```python
from build123d import *

# Parameters (mm, degrees)
SKETCH_1_W                  = 66
SKETCH_1_H                  = 56
EXTRUDE_1_DEPTH             = 2
SKETCH_2_R                  = 1.6
CUT_EXTRUDE_1_DEPTH         = 2
PATTERN_LINEAR_1_COUNT      = 2
PATTERN_LINEAR_1_PITCH      = 50
PATTERN_LINEAR_1_COUNT_DIR2 = 2
PATTERN_LINEAR_1_PITCH_DIR2 = 40
SKETCH_4_R                  = 1.6
CUT_EXTRUDE_2_DEPTH         = 2
SKETCH_5_W                  = 18
SKETCH_5_H                  = 14
CUT_EXTRUDE_3_DEPTH         = 2
SKETCH_7_W                  = 18
SKETCH_7_H                  = 14
CUT_EXTRUDE_4_DEPTH         = 2
SKETCH_8_W                  = 12.2
SKETCH_8_H                  = 6.6
CUT_EXTRUDE_5_DEPTH         = 2


with BuildPart() as part:
    # 草图1 → 凸台-拉伸1 (new body)
    with BuildSketch(Plane(origin=(0, 0, 0), x_dir=(1, 0, 0), z_dir=(0, 1, 0))):
        Rectangle(SKETCH_1_W, SKETCH_1_H)
    extrude(amount=EXTRUDE_1_DEPTH)

    # 草图2 → 切除-拉伸1 (cut)
    with BuildSketch(Plane(origin=(0, 2, 0), x_dir=(1, 0, 0), z_dir=(0, 1, 0))):
        with Locations(Location((-25, 20, 0), (0, 0, 270))):
            Circle(SKETCH_2_R)
    cut_extrude_1 = extrude(amount=-CUT_EXTRUDE_1_DEPTH, mode=Mode.SUBTRACT)

    # 阵列(线性)1: Cut-Extrude 1 2 × 2
    with Locations(*[(i * PATTERN_LINEAR_1_PITCH, 0, j * PATTERN_LINEAR_1_PITCH_DIR2) for i in range(PATTERN_LINEAR_1_COUNT) for j in range(PATTERN_LINEAR_1_COUNT_DIR2) if (i, j) != (0, 0)]):
        add(cut_extrude_1, mode=Mode.SUBTRACT)

    # 草图4 → 切除-拉伸2 (cut)
    with BuildSketch(Plane.XZ):
        with Locations(Location((-17.49998476, 20.00007874, 0), (0, 0, 270))):
            Circle(SKETCH_4_R)
        with Locations(Location((-7.49996444, 20.00007874, 0), (0, 0, 270))):
            Circle(SKETCH_4_R)
        with Locations(Location((2.49985522, 19.999735839, 0), (0, 0, 270))):
            Circle(SKETCH_4_R)
    extrude(amount=-CUT_EXTRUDE_2_DEPTH, mode=Mode.SUBTRACT)

    # 草图5 → 切除-拉伸3 (cut)
    with BuildSketch(Plane.XZ):
        with Locations((24, 0)):
            Rectangle(SKETCH_5_W, SKETCH_5_H)
    extrude(amount=-CUT_EXTRUDE_3_DEPTH, mode=Mode.SUBTRACT)

    # 草图7 → 切除-拉伸4 (cut)
    with BuildSketch(Plane.XZ):
        with Locations((-24, -7.5)):
            Rectangle(SKETCH_7_W, SKETCH_7_H)
    extrude(amount=-CUT_EXTRUDE_4_DEPTH, mode=Mode.SUBTRACT)

    # 草图8 → 切除-拉伸5 (cut)
    with BuildSketch(Plane(origin=(0, 2, 0), x_dir=(1, 0, 0), z_dir=(0, 1, 0))):
        with Locations((-12.4999746, 19.599995025)):
            Rectangle(SKETCH_8_W, SKETCH_8_H)
    extrude(amount=-CUT_EXTRUDE_5_DEPTH, mode=Mode.SUBTRACT)


solid = part.part
```
Input: part model. Units: mm. Frame: model coordinates. A direction names the side the tool comes from. Give positions to 0.01 mm unless a question says otherwise; leave off trailing zeros. Order: outer loops, then holes, each group sorted by start corner. A loop starts at its lowest first (then second) coordinate and runs counter-clockwise, first axis right, second up.
1. Cut plane A-A (x = -25). Return loops of the section in (y, z).
Computed:
outline: (0, -28) - (2, -28) - (2, -21.6) - (0, -21.6) - close; (0, -18.4) - (2, -18.4) - (2, -14.5) - (0, -14.5) - close; (0, -0.5) - (2, -0.5) - (2, 18.4) - (0, 18.4) - close; (0, 21.6) - (2, 21.6) - (2, 28) - (0, 28) - close
2. Cut plane C-C (z = -20). Return loops of the section in (x, y), and give its area (3 significant figures).
Computed:
outline: (-33, 0) - (-26.6, 0) - (-26.6, 2) - (-33, 2) - close; (-23.4, 0) - (-18.6, 0) - (-18.6, 2) - (-23.4, 2) - close; (-6.4, 0) - (23.4, 0) - (23.4, 2) - (-6.4, 2) - close; (26.6, 0) - (33, 0) - (33, 2) - (26.6, 2) - close
area: 94.8 mm2
3. Set-up query: faces 1 (the face through (-13, 1, -22.9)), 2 (the face through (-33, 1, 14)), 3 (the face through (33, 1, 18)), 4 (the face through (15, 1, 0)), 5 (the face through (-15, 1, -8)). Return all of +Z, -Z, +X, -X, +Y, -Y with unobstructed straight access to the full face (end or side cutting, diameter ignored); none if empty.
Computed:
face 1: +Y, -Y
face 2: +Z, -Z, -X, +Y, -Y
face 3: +Z, -Z, +X, +Y, -Y
face 4: +X, +Y, -Y
face 5: -X, +Y, -Y
4. Line query: probe 1 along Z at (x, y) = (2.5, 1.1); probe 2 along X at (y, z) = (0.6, 20); probe 3 along Z at (x, y) = (20.5, 0.9). Output: solid intervals per line, ascending.
Computed:
probe 1: z = -28 to 18.4, 21.6 to 28
probe 2: x = -33 to -26.6, -23.4 to -19.1, -15.9 to -9.1, -5.9 to 0.9, 4.1 to 23.4, 26.6 to 33
probe 3: z = -28 to -7, 7 to 28
5. Pin query (flat end, axial travel): pin 1 Ø3.5 at (x, z) = (-25, -20) entering from +Y; pin 2 Ø2.5 at (x, z) = (-7.5, 20) entering from -Y; pin 3 Ø1 at (y, z) = (1.5, 0.5) entering from +X. Return the tip coordinate at first contact, or that it passes through.
Computed:
pin 1: stops at y = 2
pin 2: passes through
pin 3: stops at x = 15
6. Cut plane B-B (z = 20). Return loops of the section in (x, y).
Computed:
outline: (-33, 0) - (-26.6, 0) - (-26.6, 2) - (-33, 2) - close; (-23.4, 0) - (-19.1, 0) - (-19.1, 2) - (-23.4, 2) - close; (-15.9, 0) - (-9.1, 0) - (-9.1, 2) - (-15.9, 2) - close; (-5.9, 0) - (0.9, 0) - (0.9, 2) - (-5.9, 2) - close; (4.1, 0) - (23.4, 0) - (23.4, 2) - (4.1, 2) - close; (26.6, 0) - (33, 0) - (33, 2) - (26.6, 2) - close
7. Cut plane D-D (x = 16). Return loops of the section in (y, z).
Computed:
outline: (0, -28) - (2, -28) - (2, -7) - (0, -7) - close; (0, 7) - (2, 7) - (2, 28) - (0, 28) - close
8. Draft query along X for faces 6 (the face through (24.03, 1.01, -21.27)), 7 (the face through (33, 1, -17)), 8 (the face through (0, 2, 0)). Return one class per face: released by +X, released by -X, zero draft, split by the parting line, or undercut.
Computed:
face 6: undercut
face 7: released by +X
face 8: zero draft
